Build history of the part. All positions in model axes, mm. A direction names the side the tool comes from. Round coordinates to 2 decimals unless told otherwise and drop trailing zeros. Write each loop counter-clockwise with the first axis right and the second up, starting at its lowest first coordinate (ties: lowest second). Pieces come first, ordered by that corner, then holes. Notation, with made-up numbers: (37.25, -16) - (72.25, -16) arc R25 cw to (72.25, 19) - close; hole circle Ø5 at (53.25, -38). An arc over 180 degrees is marked (long way). One line per question, with ' | ' between items.
from build123d import *

# Parameters (mm, degrees)
F0_R     = 11
F1_DEPTH = 40
F3_D     = 3.0625
F3_DEPTH = 25
F3_TIP   = 0.9200678229
F5_D     = 2
F5_DEPTH = 25
F5_TIP   = 0.600860619
F7_D     = 3.5
F7_DEPTH = 25
F7_TIP   = 1.0515060833


with BuildPart() as f1:
    # F0 (on Top) → F1 (new body)
    with BuildSketch(Plane.XY):
        Circle(F0_R)
    extrude(amount=F1_DEPTH)

    # F3
    with Locations(Plane(origin=(0, 0, 0), x_dir=(1, 0, 0), z_dir=(0, 0, -1))):
        with Locations((0, 0)):
            Hole(F3_D / 2, depth=F3_DEPTH)
            with Locations((0, 0, -(F3_DEPTH + F3_TIP / 2))):  # 118° drill point
                Cone(0, F3_D / 2, F3_TIP, mode=Mode.SUBTRACT)

    # F5
    with Locations(Plane.XY.offset(40)):
        with Locations((0, 5.5), (5.5, 0), (-5.5, 0), (0, -5.5)):
            Hole(F5_D / 2, depth=F5_DEPTH)
            with Locations((0, 0, -(F5_DEPTH + F5_TIP / 2))):  # 118° drill point
                Cone(0, F5_D / 2, F5_TIP, mode=Mode.SUBTRACT)

    # F7
    with Locations(Plane.XY.offset(40)):
        with Locations((-3.8890872965, 3.8890872965), (3.8890872965, 3.8890872965), (3.8890872965, -3.8890872965), (-3.8890872965, -3.8890872965)):
            Hole(F7_D / 2, depth=F7_DEPTH)
            with Locations((0, 0, -(F7_DEPTH + F7_TIP / 2))):  # 118° drill point
                Cone(0, F7_D / 2, F7_TIP, mode=Mode.SUBTRACT)


solid = f1.part
Q1. Saw through at A-A, the plane z = 7. List the corners of the cut face in (x, y), then the cut area to 3 significant figures.
Found:
outline: circle Ø22 at (0, 0); hole circle Ø3.06 at (0, 0) | area: 373 mm^2
Q2. Drill centre lines: L1, parallel to Y at x = 0, z = 26.25; L2, parallel to X at y = -4.25, z = 36.5; L3, parallel to Y at x = -2.75, z = 28. Where is each one in solid material? Low to high. Write a range as from..to.
Found:
L1: -11..-6.5, -4.5..4.5, 6.5..11 | L2: -10.15..-5.6, -2.18..2.18, 5.6..10.15 | L3: -10.65..-5.22, -2.56..2.56, 5.22..10.65
Q3. Pull direction X, two halves, no side cores. Call faces 4 (the cylindrical face through (-2.38, -10.74, 19.72)), 5 (the cylindrical face through (6.3, -0.6, 27.3)), 6 (the flat face through (0, 0, 40)): +X half, -X half, draft (parallel to the pull), parting line (faces both ways), or undercut.
Found:
face 4: parting line | face 5: undercut | face 6: draft
Q4. Which spindle directions (+Z, -Z, +X, -X, +Y, -Y) get a long thin tool onto all of the face, cutting with end or side? Do faces 1 (the flat face through (0, -2, 0)), 2 (the cylindrical face through (-0.823, -1.291, 12.675)), 3 (the cylindrical face through (-4.7, -0.6, 27.3)). Say none if no direction does.
Found:
face 1: -Z, +X, -X, +Y, -Y | face 2: -Z | face 3: +Z
Q5. Saw through at B-B, the plane z = 22.5. State how many separate pieces and enclosed holes the cut face has, then the cut area to 3 significant figures.
Found:
separate pieces: 1 | enclosed holes: 9 | area: 322 mm^2
Q6. Drop flat-ended pins along their axis: pin 1 (3 mm diameter, centred on x = 3.89, y = -3.89, fed in from -Z); pin 2 (2 mm diameter, centred on y = 3.5, z = 27, fed in from +X); pin 3 (1 mm diameter, centred on x = -1, z = 27.5, fed in from +Y); pin 4 (1.2 mm diameter, centred on x = -5.5, y = 0, fed in from +Z). Give the stop position or say it passes through.
Found:
pin 1: z = 0 | pin 2: x = 10.71 | pin 3: y = 10.99 | pin 4: z = 14.76
Q7. Saw through at D-D, the plane y = 7.25. List the corners of the cut face in (x, z), then the cut area to 3 significant figures.
Found:
outline: (-8.27, 0) - (8.27, 0) - (8.27, 40) - (-8.27, 40) - close | area: 662 mm^2
Q8. Saw through at C-C, the plane y = -7.5. List the corners of the cut face in (x, z), then the cut area to 3 significant figures.
Found:
outline: (-8.05, 0) - (8.05, 0) - (8.05, 40) - (-8.05, 40) - close | area: 644 mm^2
